The model under review builds one solid part; all positions refer to its coordinate system, in mm. A direction names the side the tool comes from. Coordinates: 2 decimals unless noted, no trailing zeros. Write each loop counter-clockwise with the first axis right and the second up, starting at its lowest first coordinate (ties: lowest second). Pieces come first, ordered by that corner, then holes. Notation, with made-up numbers: M 40.5,33 L 62.5,33 A35 cw 62.5,72 Z; hole C -7,69.25 d1. An arc over 180 degrees is marked long. Answer as a JSON object with one key per item and string values.
```python
from build123d import *

# Parameters (mm, degrees)
SKETCH1_W              = 9
SKETCH1_H              = 9
SKETCH1_W_2            = 2.5
SKETCH1_H_2            = 6
BOSS_EXTRUDE1_DEPTH    = 8
SKETCH2_W              = 9
SKETCH2_H              = 9
BOSS_EXTRUDE2_DEPTH    = 20
SKETCH3_R              = 2.125
CUT_EXTRUDE2_DEPTH     = 13
CUT_EXTRUDE4_START     = -6.363961131
CUT_EXTRUDE4_OUTLINE_R = 0.9
CUT_EXTRUDE4_DEPTH     = 12.727922262


# Read off the part's stored shape, not the designer's step: Cut-Extrude4
with BuildPart() as part:
    # Sketch1 → Boss-Extrude1 (new body)
    with BuildSketch(Plane(origin=(0, 0, 0), x_dir=(1, 0, 0), z_dir=(0, 1, 0))):
        Rectangle(SKETCH1_W, SKETCH1_H)
        with Locations((-1.75, 0)):
            Rectangle(SKETCH1_W_2, SKETCH1_H_2, mode=Mode.SUBTRACT)
        with Locations((1.75, 0)):
            Rectangle(SKETCH1_W_2, SKETCH1_H_2, mode=Mode.SUBTRACT)
    extrude(amount=BOSS_EXTRUDE1_DEPTH)

    # Sketch2 → Boss-Extrude2 (add)
    with BuildSketch(Plane(origin=(0, 8, 0), x_dir=(1, 0, 0), z_dir=(0, 1, 0))):
        Rectangle(SKETCH2_W, SKETCH2_H)
    extrude(amount=BOSS_EXTRUDE2_DEPTH)

    # Sketch3 → Cut-Extrude2 (cut)
    with BuildSketch(Plane(origin=(0, 28, 0), x_dir=(1, 0, 0), z_dir=(0, 1, 0))):
        with Locations(Location((0, 0, 0), (0, 0, 270))):
            Circle(SKETCH3_R)
    extrude(amount=-CUT_EXTRUDE2_DEPTH, mode=Mode.SUBTRACT)

    # Cut-Extrude4 outline → Cut-Extrude4 (cut)
    with BuildSketch(Plane(origin=(0, 0, 0), x_dir=(0.707106781186548, 0, -0.707106781186547), z_dir=(0.707106781186547, 0, 0.707106781186548)).offset(CUT_EXTRUDE4_START)):
        with Locations((0, 12)):
            Circle(CUT_EXTRUDE4_OUTLINE_R)
    extrude(amount=CUT_EXTRUDE4_DEPTH, mode=Mode.SUBTRACT)


solid = part.part
```
(1) Add section B-B on y = 1.5. Give the boundary of the cut face in (x, z).
Results list:
{"outline": "M -4.5,-4.5 L 4.5,-4.5 L 4.5,4.5 L -4.5,4.5 Z; hole M -3,-3 L -0.5,-3 L -0.5,3 L -3,3 Z; hole M 0.5,-3 L 3,-3 L 3,3 L 0.5,3 Z"}
(2) For pin 1 Ø0.8 at (x, z) = (2, 0.5) entering from -Y, flat-tipped, find the tip position at first contact; note if it passes through.
Results list:
{"pin 1": "y = 8"}
(3) Draft analysis for pull direction Z (two halves, no side actions). For faces 1 (the face through (-4.5, 14, 0)), 2 (the face through (-3, 4, 0)), 3 (the face through (0, 14, -4.5)), state which applies: released by +Z, released by -Z, zero draft, split by the parting line, or undercut.
Results list:
{"face 1": "zero draft", "face 2": "undercut", "face 3": "released by -Z"}
(4) Add section A-A on y = 26. Give the boundary of the cut face in (x, z) (3 decimals).
Results list:
{"outline": "M -4.5,-4.5 L 4.5,-4.5 L 4.5,4.5 L -4.5,4.5 Z; hole C 0,0 d4.25"}
(5) For faces 4 (the face through (0.5, 4, 0)), 5 (the face through (-2.1, 28, 0.9)), 6 (the face through (2.107, 21.591, -0.277)), list the 3-axis set-ups (+Z, -Z, +X, -X, +Y, -Y) from which the entire face can be reached by the end or side of a thin tool; tool diameter is ignored.
Results list:
{"face 4": "-Y", "face 5": "+Z, -Z, +X, -X, +Y", "face 6": "+Y"}
(6) Wall thickness on line 1 along X through (y, z) = (6, -0.5); line 2 along X through (y, z) = (15.75, 0) (3 decimals); line 3 along Y through (x, z) = (-2.75, -2.75): over which ranges is each line inside the solid? List them lowest first. Write a range as from..to.
Results list:
{"line 1": "-4.5..-3, -0.5..0.5, 3..4.5", "line 2": "-4.5..-2.125, 2.125..4.5", "line 3": "8..11.1, 12.9..28"}
